Autodesk Inventor part; units mm, degrees
ref_plane "작업 평면1" through (0, 0, -68.75) normal (0, 0, 1) x (1, 0, 0)
ref_plane "YZ Plane" through (0, 0, 0) normal (1, 0, 0) x (0, 1, 0)
ref_plane "XZ Plane" through (0, 0, 0) normal (0, 1, 0) x (-1, 0, 0)
sketch "스케치1" plane through (0, 0, 0) normal (0, 0, 1) x (1, 0, 0)
  line L0 (-7.5, -15) -> (7.5, -15)
  line L1 (7.5, -15) -> (7.5, 15)
  line L2 (7.5, 15) -> (-7.5, 15)
  line L3 (-7.5, 15) -> (-7.5, -15)
  point P0 (0, 0)
  dimension "d0" = 15
  dimension "d1" = 30
  dimension "d2" = 15
  dimension "d3" = 7.5
extrude "돌출1" add sketch "스케치1" against normal blind 37.5
sketch "스케치2" plane through (0, 0, -37.5) normal (0, 0, -1) x (-1, 0, 0)
  line L0 (5, 11.25) -> (-5, 11.25)
  line L1 (-5, 11.25) -> (-5, -11.25)
  line L2 (-5, -11.25) -> (5, -11.25)
  line L3 (5, -11.25) -> (5, 11.25)
  line L4 (5, 11.25) -> (-5, -11.25) construction
  line L5 (-5, 11.25) -> (5, -11.25) construction
  line L6 (-4, -10) -> (4, -10)
  line L7 (4, -10) -> (4, 10)
  line L8 (4, 10) -> (-4, 10)
  line L9 (-4, 10) -> (-4, -10)
  line L10 (-4, -10) -> (4, 10) construction
  line L11 (4, -10) -> (-4, 10) construction
  point P0 (0, 0)
  dimension "d6" = 10
  dimension "d7" = 22.5
  dimension "d10" = 8
  dimension "d11" = 20
extrude "돌출2" add sketch "스케치2" along normal blind 100
sketch "스케치3" plane through (0, 0, 0) normal (0, 0, 1) x (1, 0, 0)
  line L0 (-3.95, -5) -> (3.95, -5)
  line L1 (3.95, -5) -> (3.95, 5)
  line L2 (3.95, 5) -> (-3.95, 5)
  line L3 (-3.95, 5) -> (-3.95, -5)
  line L4 (-3.95, -5) -> (3.95, 5) construction
  line L5 (3.95, -5) -> (-3.95, 5) construction
  point P0 (0, 0)
  dimension "d12" = 7.9
  dimension "d13" = 10
extrude "돌출3" add sketch "스케치3" along normal blind 15
sketch "스케치4" plane through (3.95, -5, 0) normal (1, 0, 0) x (0, 0, -1)
  circle A0 centre (-10, 5) radius 2.1
  line L0 (0, 0) -> (-15, 0)
  line L1 (-15, 0) -> (-15, 10)
  point P0 (0, 5)
  dimension "d16" = 4.2
  dimension "d17" = 5
  dimension "d18" = 5
extrude "돌출4" cut sketch "스케치4" against normal blind 15
sketch "스케치5" plane through (0, 0, -137.5) normal (0, 0, -1) x (-1, 0, 0)
  line L0 (-5, 11.25) -> (5, 11.25)
  line L1 (5, -11.25) -> (-5, -11.25)
  line L2 (5, 11.25) -> (-5, 11.25)
  line L3 (-5, 11.25) -> (-5, -11.25)
  line L4 (-5, -11.25) -> (5, -11.25)
  line L5 (5, -11.25) -> (5, 11.25)
  point P0 (7.5, 15)
  point P1 (-7.5, -15)
extrude "돌출5" add sketch "스케치5" against normal blind 2
ref_plane "작업 평면1" through (0, 0, -68.75) normal (0, 0, 1) x (1, 0, 0)
mirror "미러1" about plane through (0, 0, -68.75) normal (0, 0, 1) of "돌출3"
mirror "미러2" about plane through (0, 0, -68.75) normal (0, 0, 1) of "돌출4"
fillet "모깎기1" radius 4 4 edges at (0, -5, 15) (0, 5, 15) (0, -5, -152.5) (0, 5, -152.5)
properties part number "각도조절 액추에이터_최대" material "철, 가단"
Part model, mm, in its own coordinate system. A direction names the side the tool comes from. Round coordinates to 2 decimals unless told otherwise and drop trailing zeros. Loops run counter-clockwise (first coordinate to the right, second up) from the corner with the lowest first, then second, coordinate; pieces in that order, holes last. Notation, with made-up numbers: (-6.75, -23) - (49.25, -23) arc R25 ccw to (49.25, -11) - close; hole circle Ø10 at (-21.5, 84). An arc over 180 degrees is marked (long way). Answer as a JSON object with one key per item and string values.
Item 1: Tool access for faces 1 (the face through (0, 11.25, -87)), 2 (the face through (0, 5, 5)), 3 (the face through (0, 0, -37.5)): list every direction of +Z, -Z, +X, -X, +Y, -Y with a clear straight run to the whole face (end or side of a thin tool).
Output:
{"face 1": "-Z, +X, -X, +Y", "face 2": "+Z, +X, -X, +Y", "face 3": "none"}
Item 2: Wall check: L1, parallel to X at y = -7.75, z = -131; L2, parallel to Z at x = 3.5, y = -5.25; L3, parallel to Y at x = 1.75, z = 10. Give the ranges that are in metal, low to high.
Output:
{"L1": "-5 to -4, 4 to 5", "L2": "-137.5 to -135.5, -37.5 to 0", "L3": "-5 to -2.1, 2.1 to 5"}
Item 3: Pin check, flat tips, straight feed: pin 1 (2 mm diameter, centred on x = 0, y = -1.5, fed in from +Z); pin 2 (5 mm diameter, centred on x = -2, y = 11, fed in from +Z); pin 3 (1 mm diameter, centred on x = -1, y = 8.5, fed in from -Z); pin 4 (8 mm diameter, centred on x = 0.5, z = -111, fed in from +Y). Stop position of each tip, or through.
Output:
{"pin 1": "z = 15", "pin 2": "z = 0", "pin 3": "z = -137.5", "pin 4": "y = 11.25"}
Item 4: Band-saw the part on C-C on z = -86.5. List the corners of the cut face in (x, y).
Output:
{"outline": "(-5, -11.25) - (5, -11.25) - (5, 11.25) - (-5, 11.25) - close; hole (-4, -10) - (4, -10) - (4, 10) - (-4, 10) - close"}
Item 5: Band-saw the part on B-B on y = -7.25. List the corners of the cut face in (x, z).
Output:
{"outline": "(-7.5, -37.5) - (-5, -37.5) - (-5, -137.5) - (5, -137.5) - (5, -37.5) - (7.5, -37.5) - (7.5, 0) - (-7.5, 0) - close; hole (-4, -135.5) - (4, -135.5) - (4, -37.5) - (-4, -37.5) - close"}
Item 6: Pull direction X, two halves, no side cores. Call faces 4 (the face through (0, 10, -86)), 5 (the face through (3.95, 0, -145)), 6 (the face through (-5, 0, -87)): pulls with the +X half, pulls with the -X half, needs draft (parallel to the pull), parting line crosses it, or undercut.
Output:
{"face 4": "undercut", "face 5": "pulls with the +X half", "face 6": "pulls with the -X half"}
Item 7: Band-saw the part on A-A on x = -1.5. List the corners of the cut face in (y, z), plus the area to 3 significant figures.
Output:
{"outline": "(-15, -37.5) - (-11.25, -37.5) - (-11.25, -137.5) - (-5, -137.5) - (-5, -148.5) arc R4 ccw to (-1, -152.5) - (1, -152.5) arc R4 ccw to (5, -148.5) - (5, -137.5) - (11.25, -137.5) - (11.25, -37.5) - (15, -37.5) - (15, 0) - (5, 0) - (5, 11) arc R4 ccw to (1, 15) - (-1, 15) arc R4 ccw to (-5, 11) - (-5, 0) - (-15, 0) - close; hole (-10, -135.5) - (10, -135.5) - (10, -37.5) - (-10, -37.5) - close; hole circle Ø4.2 at (0, -147.5); hole circle Ø4.2 at (0, 10)", "area": "1,670 mm2"}
